from build123d import *

# Parameters (mm, degrees)
SKETCH1_W           = 66
SKETCH1_H           = 41
BOSS_EXTRUDE1_DEPTH = 4
SKETCH3_W           = 66
SKETCH3_H           = 41
SKETCH3_W_2         = 61
SKETCH3_H_2         = 36
BOSS_EXTRUDE3_DEPTH = 24
SKETCH2_R           = 0.9
BOSS_EXTRUDE4_DEPTH = 16
SKETCH4_R           = 2
BOSS_EXTRUDE5_DEPTH = 6
SKETCH5_W           = 12
SKETCH5_H           = 6
CUT_EXTRUDE1_DEPTH  = 6
FILLET2_R           = 2
FILLET3_R           = 2
SKETCH6_W           = 16
SKETCH6_H           = 9
CUT_EXTRUDE2_DEPTH  = 6


with BuildPart() as part:
    # Sketch1 → Boss-Extrude1 (new body)
    with BuildSketch(Plane(origin=(0, 0, 0), x_dir=(1, 0, 0), z_dir=(0, 1, 0))):
        with Locations((25.5, 13)):
            Rectangle(SKETCH1_W, SKETCH1_H)
    extrude(amount=BOSS_EXTRUDE1_DEPTH)

    # Sketch3 → Boss-Extrude3 (add)
    with BuildSketch(Plane(origin=(0, 4, 0), x_dir=(1, 0, 0), z_dir=(0, 1, 0))):
        with Locations((25.5, 13)):
            Rectangle(SKETCH3_W, SKETCH3_H)
        with Locations((25.5, 13)):
            Rectangle(SKETCH3_W_2, SKETCH3_H_2, mode=Mode.SUBTRACT)
    extrude(amount=BOSS_EXTRUDE3_DEPTH)

    # Sketch2 → Boss-Extrude4 (add)
    with BuildSketch(Plane(origin=(0, 4, 0), x_dir=(1, 0, 0), z_dir=(0, 1, 0))):
        with Locations(Location((1.8, 24.2, 0), (0, 0, 270))):
            Circle(SKETCH2_R)
        with Locations(Location((1.8, 1.8, 0), (0, 0, 90))):
            Circle(SKETCH2_R)
        with Locations(Location((49.2, 1.8, 0), (0, 0, 270))):
            Circle(SKETCH2_R)
        with Locations(Location((49.2, 24.2, 0), (0, 0, 90))):
            Circle(SKETCH2_R)
    extrude(amount=BOSS_EXTRUDE4_DEPTH)

    # Sketch4 → Boss-Extrude5 (add)
    with BuildSketch(Plane(origin=(0, 4, 0), x_dir=(1, 0, 0), z_dir=(0, 1, 0))):
        with Locations(Location((1.8, 24.2, 0), (0, 0, 270))):
            Circle(SKETCH4_R)
        with Locations(Location((1.8, 1.8, 0), (0, 0, 90))):
            Circle(SKETCH4_R)
        with Locations(Location((49.2, 1.8, 0), (0, 0, 270))):
            Circle(SKETCH4_R)
        with Locations(Location((49.2, 24.2, 0), (0, 0, 90))):
            Circle(SKETCH4_R)
    extrude(amount=BOSS_EXTRUDE5_DEPTH)

    # Sketch5 → Cut-Extrude1 (cut)
    with BuildSketch(Plane(origin=(58.5, 0, 0), x_dir=(0, 0, -1), z_dir=(1, 0, 0))):
        with Locations((10, 13)):
            Rectangle(SKETCH5_W, SKETCH5_H)
    extrude(amount=-CUT_EXTRUDE1_DEPTH, mode=Mode.SUBTRACT)

    # Fillet2
    fillet2_edges = [part.edges().sort_by_distance(p)[0] for p in [
        (-7.5, 14, 7.5),
        (-7.5, 14, -33.5),
        (58.5, 14, -33.5),
        (58.5, 14, 7.5),
    ]]
    fillet(fillet2_edges, radius=FILLET2_R)

    # Fillet3
    fillet3_edges = [part.edges().sort_by_distance(p)[0] for p in [
        (57.25, 16, -4),
        (57.25, 16, -16),
    ]]
    fillet(fillet3_edges, radius=FILLET3_R)

    # Sketch6 → Cut-Extrude2 (cut)
    with BuildSketch(Plane.XY.offset(7.5)):
        with Locations((33, 19.5)):
            Rectangle(SKETCH6_W, SKETCH6_H)
    extrude(amount=-CUT_EXTRUDE2_DEPTH, mode=Mode.SUBTRACT)


solid = part.part
Source: CAD feature listing. Evaluate the final solid. Frame: model axes, mm. A direction names the side the tool comes from. Round coordinates to 2 decimals unless told otherwise and drop trailing zeros. Loops run counter-clockwise (first coordinate to the right, second up) from the corner with the lowest first, then second, coordinate; pieces in that order, holes last. Notation, with made-up numbers: (11, -14.5) - (29, -14.5) arc R28 cw to (29, 16.5) - close; hole circle Ø8 at (19, 75.25). An arc over 180 degrees is marked (long way). Write item = value, one per line. Start each with the question number.
(1) Ray query, line 1 along X through (y, z) = (5.25, -22); line 2 along Z through (x, y) = (-1, 25.5); line 3 along Y through (x, z) = (0.5, -26). Return the intervals inside material, ascending. Write a range as from..to.
(2) Set-up query: faces 5 (the face through (25, 0, -13)), 6 (the face through (-6.93, 14.2, 6.9)), 7 (the face through (25, 19, 6)), 8 (the face through (25, 13, 5)), 9 (the face through (57, 12, -16)). Return all of +Z, -Z, +X, -X, +Y, -Y with unobstructed straight access to the full face (end or side cutting, diameter ignored); none if empty.
(3) Pin query (flat end, axial travel): pin 1 (2 mm diameter, centred on y = 20.5, z = 6.5, fed in from +X); pin 2 (3 mm diameter, centred on x = 1, z = -2, fed in from +Y); pin 3 (0.8 mm diameter, centred on y = 21.5, z = 6.5, fed in from -X). Return the tip coordinate at first contact, or that it passes through.
(4) Section query D-D, the plane x = 49.2. Output: boundary loops of the cut face in (y, z), plus the area to 3 significant figures.
(5) Section query C-C, the plane z = -28.5. Output: boundary loops of the cut face in (x, y).
(6) Pull-direction query (Z, two-part tool) for faces 1 (the face through (58.5, 17, -13)), 2 (the face through (1.002, 14.93, -23.785)), 3 (the face through (25, 16, -31)), 4 (the face through (57.9, 14.2, 6.93)); classes: +Z half, -Z half, draft (parallel to the pull), parting line (faces both ways), or undercut.
(7) Section query A-A, the plane y = 17.25. Output: boundary loops of the cut face in (x, z).
(8) Section query B-B, the plane x = 33. Output: boundary loops of the cut face in (y, z), plus the area to 4 significant figures.
Conclusion:
q1.line_1 = -7.5..-5, 56..58.5
q1.line_2 = -33.5..-31, 5..7.5
q1.line_3 = 0..4
q2.face_5 = +Z, -Z, +X, -X, -Y
q2.face_6 = +Z, -X, +Y, -Y
q2.face_7 = +Z
q2.face_8 = +Y
q2.face_9 = +X
q3.pin_1 = 58.5
q3.pin_2 = 20
q3.pin_3 = -7.41
q4.outline = (0, -33.5) - (28, -33.5) - (28, -31) - (4, -31) - (4, -26.2) - (10, -26.2) - (10, -25.1) - (20, -25.1) - (20, -23.3) - (10, -23.3) - (10, -22.2) - (4, -22.2) - (4, -3.8) - (10, -3.8) - (10, -2.7) - (20, -2.7) - (20, -0.9) - (10, -0.9) - (10, 0.2) - (4, 0.2) - (4, 5) - (28, 5) - (28, 7.5) - (0, 7.5) - close
q4.area = 368 mm2
q5.outline = (-7.5, 0) - (58.5, 0) - (58.5, 28) - (56, 28) - (56, 4) - (-5, 4) - (-5, 28) - (-7.5, 28) - close
q6.face_1 = draft
q6.face_2 = undercut
q6.face_3 = undercut
q6.face_4 = +Z half
q7.outline = (-7.5, -31.5) arc R2 ccw to (-5.5, -33.5) - (56.5, -33.5) arc R2 ccw to (58.5, -31.5) - (58.5, 5.5) arc R2 ccw to (56.5, 7.5) - (41, 7.5) - (41, 5) - (56, 5) - (56, -31) - (-5, -31) - (-5, 5) - (25, 5) - (25, 7.5) - (-5.5, 7.5) arc R2 ccw to (-7.5, 5.5) - close; circle Ø1.8 at (1.8, -24.2); circle Ø1.8 at (1.8, -1.8); circle Ø1.8 at (49.2, -24.2); circle Ø1.8 at (49.2, -1.8)
q8.outline = (0, -33.5) - (28, -33.5) - (28, -31) - (4, -31) - (4, 5) - (15, 5) - (15, 7.5) - (0, 7.5) - close; (24, 5) - (28, 5) - (28, 7.5) - (24, 7.5) - close
q8.area = 261.5 mm2
